Autodesk Inventor part; units mm, degrees
ref_plane "Work Plane1" through (-340, 0, -30) normal (-1, 0, 0) x (0, -1, 0)
ref_plane "YZ Plane" through (0, 0, 0) normal (1, 0, 0) x (0, 1, 0)
ref_plane "XZ Plane" through (0, 0, 0) normal (0, 1, 0) x (-1, 0, 0)
sketch "Sketch1" plane through (0, 0, 0) normal (0, 1, 0) x (-1, 0, 0)
  line L0 (370, 0) -> (-370, 0) construction
  line L1 (340, 30) -> (-340, 30)
  line L2 (-340, -30) -> (340, -30)
  arc A0 (340, -30) -> (340, 30) centre (340, 0) ccw
  arc A1 (-340, 30) -> (-340, -30) centre (-340, 0) ccw
  point P0 (0, 0)
  point P1 (0, 0)
  point P2 (-370, 0)
  point P3 (370, 0)
  dimension "d2" = 60
  dimension "d7" = 680
ref_plane "Work Plane1" through (-340, 0, -30) normal (-1, 0, 0) x (0, -1, 0)
sketch "Sketch2" plane through (-340, 0, -30) normal (-1, 0, 0) x (0, -1, 0)
  line L0 (-120, 0) -> (120, 0)
  line L1 (120, 0) -> (120, -2)
  line L2 (120, -2) -> (-120, -2)
  line L3 (-120, -2) -> (-120, 0)
  line L4 (-120, 0) -> (120, -2) construction
  line L5 (120, 0) -> (-120, -2) construction
  line L6 (0, 60) -> (0, 0)
  point P0 (0, 30)
  dimension "d3" = 240
  dimension "d4" = 2
sweep "Sweep1" add profiles "Sketch2" path "Sketch1"
properties part number "HCMUTE-CDT23-BELT_BTC" material "PVC, Unplasticized"
Verification items for the finished model (mm, model axes). A direction names the side the tool comes from. Round coordinates to 2 decimals unless told otherwise and drop trailing zeros. Loops run counter-clockwise (first coordinate to the right, second up) from the corner with the lowest first, then second, coordinate; pieces in that order, holes last. Notation, with made-up numbers: (5.25, -24) - (42.25, -24) arc R12 cw to (42.25, -8) - close; hole circle Ø10 at (20.5, 12.25). An arc over 180 degrees is marked (long way). Answer in a Markdown table with one row per item. Add a question column.
Q1. Section check C-C on y = -90.5. Enter the section's corners in (x, z), plus the area to 3 significant figures.
Q2. Tool access check on faces 1 (the face through (371.992, -1.68, -0.704)), 2 (the face through (-5, -2, -30)). Record the directions out of +Z, -Z, +X, -X, +Y, -Y that give a thin tool (end or side, any length) a straight path to the whole face; none if there is none.
Q3. Gauge pin test, flat ends, axial feed: pin 1 (6 mm diameter, centred on y = 55, z = 1.5, fed in from -X); pin 2 (4 mm diameter, centred on y = -13, z = -12, fed in from -X). Record the tip position at first contact, or that the pin passes through.
Q4. Material ranges on line 1 (Z direction, x = 117, y = -34.5); line 2 (X direction, y = -59.5, z = 20.5); line 3 (X direction, y = -56, z = 0), recorded low to high.
Q5. Section check B-B on z = 0. Enter the section's corners in (x, y).
Q6. Section check A-A on x = -112.5. Enter the section's corners in (y, z).
Q7. Release check for a two-part mould opening along Z. For faces 3 (the face through (-2, -120, -31)), 4 (the face through (369.993, 1.68, 0.66)), 5 (the face through (-371.992, -1.68, 0.704)) record: pulls with the +Z half, pulls with the -Z half, needs draft (parallel to the pull), parting line crosses it, or undercut.
Found:
| question | item | result |
|---|---|---|
| 1 | outline | (-340, -32) - (340, -32) arc R32 ccw to (340, 32) - (-340, 32) arc R32 ccw to start; hole (-340, -30) - (340, -30) arc R30 ccw to (340, 30) - (-340, 30) arc R30 ccw to start |
| 1 | area | 3,110 mm² |
| 2 | face 1 | +X, +Y, -Y |
| 2 | face 2 | +Y, -Y |
| 3 | pin 1 | stops at x = -372 |
| 3 | pin 2 | stops at x = -370.4 |
| 4 | line 1 | z = -32 to -30, 30 to 32 |
| 4 | line 2 | x = -364.57 to -361.9, 361.9 to 364.57 |
| 4 | line 3 | x = -372 to -370, 370 to 372 |
| 5 | outline | (-372, -120) - (-370, -120) - (-370, 120) - (-372, 120) - close; (370, -120) - (372, -120) - (372, 120) - (370, 120) - close |
| 6 | outline | (-120, -32) - (120, -32) - (120, -30) - (-120, -30) - close; (-120, 30) - (120, 30) - (120, 32) - (-120, 32) - close |
| 7 | face 3 | needs draft |
| 7 | face 4 | undercut |
| 7 | face 5 | parting line crosses it |
